Check sheet for the drawn part. Datum: minimum x, y, z corner. Units: mm. A direction names the side the tool comes from. Coordinates: 2 decimals unless noted, no trailing zeros. Order: outer loops, then holes, each group sorted by start corner. A loop starts at its lowest first (then second) coordinate and runs counter-clockwise, first axis right, second up.
1. Cross-section at C-C (x = 2.15). Enter the section's corners in (y, z).
2. Cross-section at B-B (z = 3.5). Enter the section's corners in (x, y), then the cut area to 3 significant figures.
3. Gauge pin test, flat end, axial feed: pin 1 Ø2 at (y, z) = (2, 14.5) entering from +X. Record the tip position at first contact, or that the pin passes through.
4. Set-up check for the marked faces 5 and 6: record each of +Z, -Z, +X, -X, +Y, -Y from which the full face is reachable in a straight line by a thin tool's end or side.
5. Draft check along Y on the marked faces 1, 2, 3 and 4. Enter one of: released by +Y, released by -Y, zero draft, split by the parting line, or undercut.
6. Thickness scan on line 1 (Y direction, x = 1.25, z = 3.5); line 2 (Z direction, x = 1.2, y = 3.8); line 3 (Z direction, x = 2.55, y = 2.3). Record the ranges inside material, lowest first.
7. Cross-section at D-D (x = 3.6). Enter the section's corners in (y, z), then the cut area to 3 significant figures.
8. Cross-section at A-A (y = 2.5). Enter the section's corners in (x, z), then the cut area to 3 significant figures.
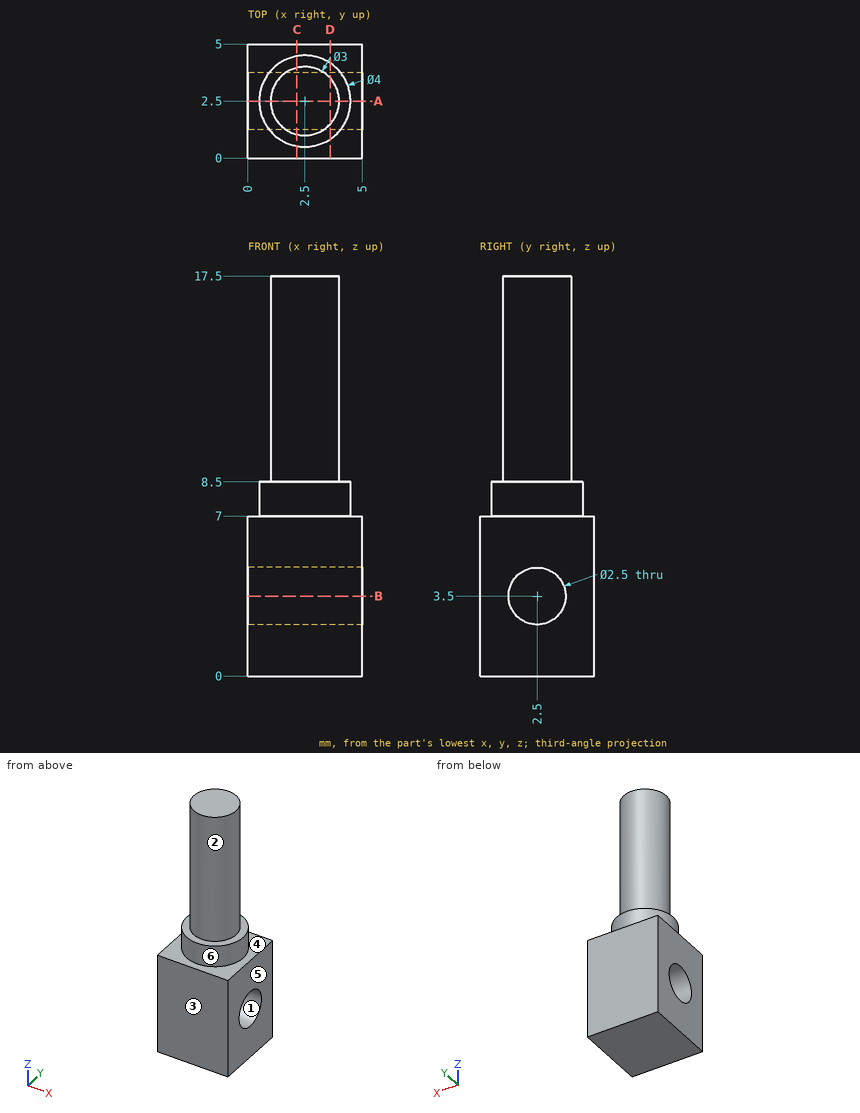
Data:
1. outline: (0, 0) - (5, 0) - (5, 7) - (4.47, 7) - (4.47, 8.5) - (3.96, 8.5) - (3.96, 17.5) - (1.04, 17.5) - (1.04, 8.5) - (0.53, 8.5) - (0.53, 7) - (0, 7) - close; hole circle Ø2.5 at (2.5, 3.5)
2. outline: (0, 0) - (5, 0) - (5, 1.25) - (0, 1.25) - close; (0, 3.75) - (5, 3.75) - (5, 5) - (0, 5) - close
2. area: 12.5 mm2
3. pin 1: stops at x = 4
4. face 5: +Z, -Z, +X, +Y, -Y
4. face 6: +Z
5. face 1: undercut
5. face 2: split by the parting line
5. face 3: released by -Y
5. face 4: zero draft
6. line 1: y = 0 to 1.25, 3.75 to 5
6. line 2: z = 0 to 8.5
6. line 3: z = 0 to 2.27, 4.73 to 17.5
7. outline: (0, 0) - (5, 0) - (5, 7) - (4.17, 7) - (4.17, 8.5) - (3.52, 8.5) - (3.52, 17.5) - (1.48, 17.5) - (1.48, 8.5) - (0.83, 8.5) - (0.83, 7) - (0, 7) - close; hole circle Ø2.5 at (2.5, 3.5)
7. area: 53.5 mm2
8. outline: (0, 0) - (5, 0) - (5, 2.25) - (0, 2.25) - close; (0, 4.75) - (5, 4.75) - (5, 7) - (4.5, 7) - (4.5, 8.5) - (4, 8.5) - (4, 17.5) - (1, 17.5) - (1, 8.5) - (0.5, 8.5) - (0.5, 7) - (0, 7) - close
8. area: 55.5 mm2
